For this review, take the finished solid that the model builds, in its own axes (mm). A direction names the side the tool comes from. Coordinates: 2 decimals unless noted, no trailing zeros. Write each loop counter-clockwise with the first axis right and the second up, starting at its lowest first coordinate (ties: lowest second). Pieces come first, ordered by that corner, then holes. Notation, with made-up numbers: (-8, -7.75) -> (-4, -7.75) arc R30 ccw to (-4, 26.25) -> close; hole circle Ø2 at (-22, 13.25). An arc over 180 degrees is marked (long way). Put each result on its own line as item: value. Start each with the question number.
Item 1: The part is to be moulded in two halves that separate along X. For faces 3 (the flat face through (-1, -37.3, 113)), 4 (the flat face through (-1, 37.3, 113)), 5 (the flat face through (-37.5, -28.5, 228.6)), 6 (the flat face through (-38.1, -1, 113)), say which applies: +X half, -X half, draft (parallel to the pull), parting line (faces both ways), or undercut.
Item 2: Insertion check: P1, Ø0.9, axis at x = 38, y = -1, coming from the +Z side; P2, Ø3, axis at x = -15, y = 0.5, coming from the +Z side. Each pin has a flat end and moves straight along its axis. Give the tip position at first contact, or say it passes through.
Item 3: To check wall thickness, follow L1, parallel to X at y = -9, z = 122; L2, parallel to Y at x = 0, z = 0.45. State the ranges of each line that lie inside material, in increasing order.
Item 4: For faces 1 (the flat face through (-1, -38.1, 113)), 2 (the flat face through (-37.3, -1, 113)), list the 3-axis set-ups (+Z, -Z, +X, -X, +Y, -Y) from which the entire face can be reached by the end or side of a thin tool; tool diameter is ignored.
Item 5: Consider section A-A on x = -25.5. Give the boundary of the cut face in (y, z), and give its area (3 significant figures).
Item 6: Consider section B-B on z = 198. Give the boundary of the cut face in (x, y).
```python
from build123d import *

# Parameters (mm, degrees)
F0_W     = 76.2
F0_H     = 76.2
F1_DEPTH = 228.6
F2_T     = -0.8
F3_R     = 1
F4_DEPTH = 25.4
F5_W     = 8
F5_H     = 2
F6_DEPTH = 76.201
F7_W     = 8
F7_H     = 4
F8_DEPTH = 76.201


with BuildPart() as f1:
    # F0 (on Top) → F1 (new body)
    with BuildSketch(Plane.XY):
        Rectangle(F0_W, F0_H)
    extrude(amount=F1_DEPTH)

    # F2
    f2_openings = [f1.faces().sort_by_distance(p)[0] for p in [
        (0, 0, 228.6),
    ]]
    offset(amount=F2_T, openings=f2_openings)

    # F3 (on face) → F4 (cut)
    with BuildSketch(Plane.XY.offset(0.8)):
        Circle(F3_R)
    extrude(amount=-F4_DEPTH, mode=Mode.SUBTRACT)

    # F5 (on face) → F6 (cut, through all)
    with BuildSketch(Plane.XZ.offset(38.1)):
        with Locations((0, 227.6)):
            Rectangle(F5_W, F5_H)
    extrude(amount=-F6_DEPTH, mode=Mode.SUBTRACT)

    # F7 (on face) → F8 (cut, through all)
    with BuildSketch(Plane.YZ.offset(38.1)):
        with Locations((0, 226.6)):
            Rectangle(F7_W, F7_H)
    extrude(amount=-F8_DEPTH, mode=Mode.SUBTRACT)


solid = f1.part
```
Return value:
1. face 3: undercut
1. face 4: undercut
1. face 5: draft
1. face 6: -X half
2. P1: z = 224.6
2. P2: z = 0.8
3. L1: -38.1 to -37.3, 37.3 to 38.1
3. L2: -38.1 to -1, 1 to 38.1
4. face 1: +Z, -Z, +X, -X, -Y
4. face 2: +Z
5. outline: (-38.1, 0) -> (38.1, 0) -> (38.1, 228.6) -> (37.3, 228.6) -> (37.3, 0.8) -> (-37.3, 0.8) -> (-37.3, 228.6) -> (-38.1, 228.6) -> close
5. area: 425 mm^2
6. outline: (-38.1, -38.1) -> (38.1, -38.1) -> (38.1, 38.1) -> (-38.1, 38.1) -> close; hole (-37.3, -37.3) -> (37.3, -37.3) -> (37.3, 37.3) -> (-37.3, 37.3) -> close
